Read the model definition and answer for the solid it produces. Units are mm, in the model's axes. Coordinates: 2 decimals unless noted, no trailing zeros. Loops run counter-clockwise (first coordinate to the right, second up) from the corner with the lowest first, then second, coordinate; pieces in that order, holes last. Notation, with made-up numbers: (-24, 75) -> (34, 75) arc R24 ccw to (34, 88) -> close; hole circle Ø8 at (-18, 40). An arc over 180 degrees is marked (long way). Answer as a JSON object with one key per item and string values. Group by question number.
1) A flat-ended cylindrical pin translates along its axis: P1, Ø8.5, axis at y = 62.5, z = -95, coming from the -X side. Find the tip coordinate at first contact, or state that the pin passes through.
2) Section A-A, the plane y = -62.5 is taken. Give the vertices of the cut face in (x, z) (3 decimals), plus the area to 3 significant figures.
3) Section B-B, the plane z = -95 is taken. Give the vertices of the cut face in (x, y) (3 decimals).
4) Consider probe 1 along Y at (x, z) = (0.95, -95). Determine where the line is inside the solid, lowest interval first. Write a range as [from, to].
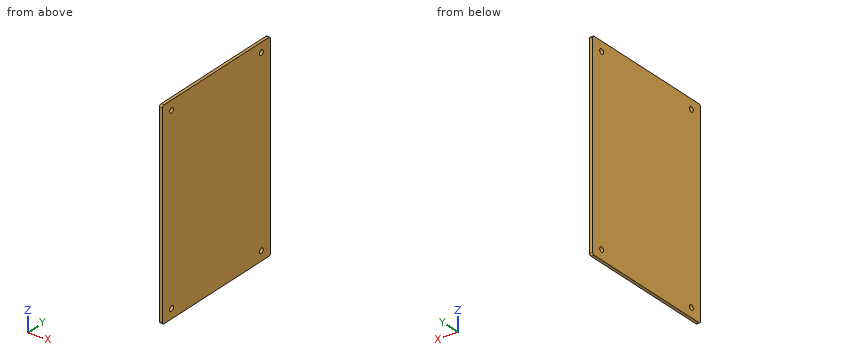
from build123d import *

# Parameters (mm, degrees)
SKETCH2_W            = 210
SKETCH2_H            = 150
BOSS_EXTRUDE1_DEPTH  = 3.175
M5_CLEARANCE_HOLE2_D = 5.3
FILLET2_R            = 2


with BuildPart() as part:
    # Sketch2 → Boss-Extrude1 (new body)
    with BuildSketch(Plane(origin=(0, 0, 0), x_dir=(0, 0, -1), z_dir=(1, 0, 0))):
        Rectangle(SKETCH2_W, SKETCH2_H)
    extrude(amount=BOSS_EXTRUDE1_DEPTH)

    # M5 Clearance Hole2 (through all)
    with Locations(Plane(origin=(3.175, 0, 0), x_dir=(0, 0, -1), z_dir=(1, 0, 0))):
        with Locations((-95, 62.5), (95, 62.5), (-95, -62.5), (95, -62.5)):
            Hole(M5_CLEARANCE_HOLE2_D / 2)

    # Fillet2
    fillet2_edges = [part.edges().sort_by_distance(p)[0] for p in [
        (1.5875, -75, -105),
        (1.5875, -75, 105),
        (1.5875, 75, 105),
        (1.5875, 75, -105),
    ]]
    fillet(fillet2_edges, radius=FILLET2_R)


solid = part.part
Determined:
{
 "1": {"P1": "x = 0"},
 "2": {"outline": "(0, -105) -> (3.175, -105) -> (3.175, -97.65) -> (0, -97.65) -> close; (0, -92.35) -> (3.175, -92.35) -> (3.175, 92.35) -> (0, 92.35) -> close; (0, 97.65) -> (3.175, 97.65) -> (3.175, 105) -> (0, 105) -> close", "area": "633 mm²"},
 "3": {"outline": "(0, -75) -> (3.175, -75) -> (3.175, -65.15) -> (0, -65.15) -> close; (0, -59.85) -> (3.175, -59.85) -> (3.175, 59.85) -> (0, 59.85) -> close; (0, 65.15) -> (3.175, 65.15) -> (3.175, 75) -> (0, 75) -> close"},
 "4": {"probe 1": "[-75, -65.15], [-59.85, 59.85], [65.15, 75]"}
}
